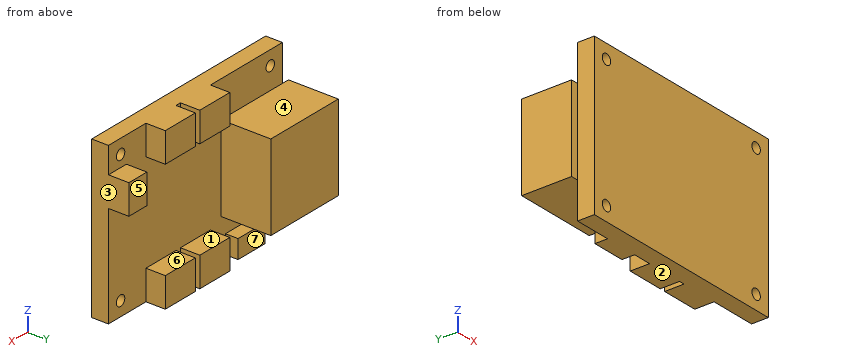
from build123d import *

# Parameters (mm, degrees)
SKETCH1_W           = 58
SKETCH1_H           = 42.5
SKETCH1_R           = 1.4
BOSS_EXTRUDE1_DEPTH = 4.5
SKETCH2_W           = 20.5
SKETCH2_H           = 23
SKETCH2_W_2         = 2
BOSS_EXTRUDE2_DEPTH = 13.4
SKETCH2_3_W         = 10
SKETCH2_3_H         = 8
BOSS_EXTRUDE3_DEPTH = 5.2
SKETCH2_4_W         = 6
SKETCH2_4_H         = 8
BOSS_EXTRUDE4_DEPTH = 5.5
SKETCH2_5_W         = 9
SKETCH2_5_H         = 5
BOSS_EXTRUDE5_DEPTH = 3.4


with BuildPart() as part:
    # Sketch1 → Boss-Extrude1 (new body)
    with BuildSketch(Plane(origin=(0, 0, 0), x_dir=(1, 0, 0), z_dir=(0, 1, 0))):
        Rectangle(SKETCH1_W, SKETCH1_H)
        with Locations(Location((-24.95, 17.4, 0), (0, 0, 270))):
            Circle(SKETCH1_R, mode=Mode.SUBTRACT)
        with Locations(Location((24.95, 17.4, 0), (0, 0, 90))):
            Circle(SKETCH1_R, mode=Mode.SUBTRACT)
        with Locations(Location((24.95, -17.4, 0), (0, 0, 270))):
            Circle(SKETCH1_R, mode=Mode.SUBTRACT)
        with Locations(Location((-24.95, -17.4, 0), (0, 0, 90))):
            Circle(SKETCH1_R, mode=Mode.SUBTRACT)
    extrude(amount=BOSS_EXTRUDE1_DEPTH)

    # Sketch2 → Boss-Extrude2 (add)
    with BuildSketch(Plane(origin=(0, 4.5, 0), x_dir=(1, 0, 0), z_dir=(0, 1, 0))):
        with Locations((-18.75, 0)):
            Rectangle(SKETCH2_W, SKETCH2_H)
        with Locations((-30, 0)):
            Rectangle(SKETCH2_W_2, SKETCH2_H)
    extrude(amount=BOSS_EXTRUDE2_DEPTH)

    # Sketch2_3 → Boss-Extrude3 (add)
    with BuildSketch(Plane(origin=(0, 4.5, 0), x_dir=(1, 0, 0), z_dir=(0, 1, 0))):
        with Locations((0, 17.25)):
            Rectangle(SKETCH2_3_W, SKETCH2_3_H)
        with Locations((11.5, 17.25)):
            Rectangle(SKETCH2_3_W, SKETCH2_3_H)
        with Locations((0, -17.25)):
            Rectangle(SKETCH2_3_W, SKETCH2_3_H)
        with Locations((11.5, -17.25)):
            Rectangle(SKETCH2_3_W, SKETCH2_3_H)
    extrude(amount=BOSS_EXTRUDE3_DEPTH)

    # Sketch2_4 → Boss-Extrude4 (add)
    with BuildSketch(Plane(origin=(0, 4.5, 0), x_dir=(1, 0, 0), z_dir=(0, 1, 0))):
        with Locations((26, -10.25)):
            Rectangle(SKETCH2_4_W, SKETCH2_4_H)
    extrude(amount=BOSS_EXTRUDE4_DEPTH)

    # Sketch2_5 → Boss-Extrude5 (add)
    with BuildSketch(Plane(origin=(0, 4.5, 0), x_dir=(1, 0, 0), z_dir=(0, 1, 0))):
        with Locations((-14.5, 18.75)):
            Rectangle(SKETCH2_5_W, SKETCH2_5_H)
    extrude(amount=BOSS_EXTRUDE5_DEPTH)


solid = part.part
Source: CAD feature listing. Evaluate the final solid. Frame: model axes, mm. Face numbers are marked on the shaded views. A direction names the side the tool comes from. Coordinates: 2 decimals unless noted, no trailing zeros. Loops run counter-clockwise (first coordinate to the right, second up) from the corner with the lowest first, then second, coordinate; pieces in that order, holes last. Notation, with made-up numbers: M 24.5,36.5 L 38.5,36.5 A25 ccw 38.5,56.5 Z; hole C 38.25,-10 d9. An arc over 180 degrees is marked long. Answer in a Markdown table with one row per item.
Q1. Section A-A on z = 17.4. Return the cut outline in (x, y).
Answers below:
| item | result |
|---|---|
| outline | M -29,0 L -26.35,0 L -26.35,4.5 L -29,4.5 Z; M -23.55,0 L 23.55,0 L 23.55,4.5 L 16.5,4.5 L 16.5,9.7 L 6.5,9.7 L 6.5,4.5 L 5,4.5 L 5,9.7 L -5,9.7 L -5,4.5 L -23.55,4.5 Z; M 26.35,0 L 29,0 L 29,4.5 L 26.35,4.5 Z |
Q2. Set-up query: the marked faces 5, 6 and 7. Return all of +Z, -Z, +X, -X, +Y, -Y with unobstructed straight access to the full face (end or side cutting, diameter ignored); none if empty.
Answers below:
| item | result |
|---|---|
| face 5 | +Z, -Z, +X, +Y |
| face 6 | +X, -X, +Y |
| face 7 | -Z, -X, +Y |
Q3. Section B-B on x = -24.95. Return the cut outline in (y, z), plus the area to 3 significant figures.
Answers below:
| item | result |
|---|---|
| outline | M 0,-21.25 L 4.5,-21.25 L 4.5,-18.8 L 0,-18.8 Z; M 0,-16 L 4.5,-16 L 4.5,-11.5 L 17.9,-11.5 L 17.9,11.5 L 4.5,11.5 L 4.5,16 L 0,16 Z; M 0,18.8 L 4.5,18.8 L 4.5,21.25 L 0,21.25 Z |
| area | 474 mm^2 |
Q4. First-contact query: pin 1 (12 mm diameter, centred on x = 15, z = 9, fed in from +Y); pin 2 (2 mm diameter, centred on y = 2, z = -9, fed in from -X); pin 3 (5.5 mm diameter, centred on y = 8, z = 18.5, fed in from -X). Flat tips, straight axial feed; report the tip coordinate or a pass-through.
Answers below:
| item | result |
|---|---|
| pin 1 | stops at y = 9.7 |
| pin 2 | stops at x = -29 |
| pin 3 | stops at x = -5 |
Q5. Draft query along Z for the marked faces 1, 2, 3 and 4. Return one class per face: pulls with the +Z half, pulls with the -Z half, needs draft (parallel to the pull), parting line crosses it, or undercut.
Answers below:
| item | result |
|---|---|
| face 1 | undercut |
| face 2 | pulls with the -Z half |
| face 3 | needs draft |
| face 4 | pulls with the +Z half |
Q6. Section D-D on x = 9. Return the cut outline in (y, z).
Answers below:
| item | result |
|---|---|
| outline | M 0,-21.25 L 9.7,-21.25 L 9.7,-13.25 L 4.5,-13.25 L 4.5,13.25 L 9.7,13.25 L 9.7,21.25 L 0,21.25 Z |
Q7. Ray query, probe 1 along X at (y, z) = (1.3, -17.4); probe 2 along X at (y, z) = (9.5, 13.5); probe 3 along X at (y, z) = (5, 7.5). Return the intervals inside material, ascending. Write a range as from..to.
Answers below:
| item | result |
|---|---|
| probe 1 | x = -29..-26.35, -23.55..23.55, 26.35..29 |
| probe 2 | x = -5..5, 6.5..16.5, 23..29 |
| probe 3 | x = -31..-8.5, 23..29 |
Q8. Section C-C on y = 6.25. Return the cut outline in (x, z), plus the area to 4 significant figures.
Answers below:
| item | result |
|---|---|
| outline | M -31,-11.5 L -8.5,-11.5 L -8.5,11.5 L -31,11.5 Z; M -19,-21.25 L -10,-21.25 L -10,-16.25 L -19,-16.25 Z; M -5,-21.25 L 5,-21.25 L 5,-13.25 L -5,-13.25 Z; M -5,13.25 L 5,13.25 L 5,21.25 L -5,21.25 Z; M 6.5,-21.25 L 16.5,-21.25 L 16.5,-13.25 L 6.5,-13.25 Z; M 6.5,13.25 L 16.5,13.25 L 16.5,21.25 L 6.5,21.25 Z; M 23,6.25 L 29,6.25 L 29,14.25 L 23,14.25 Z |
| area | 930.5 mm^2 |
